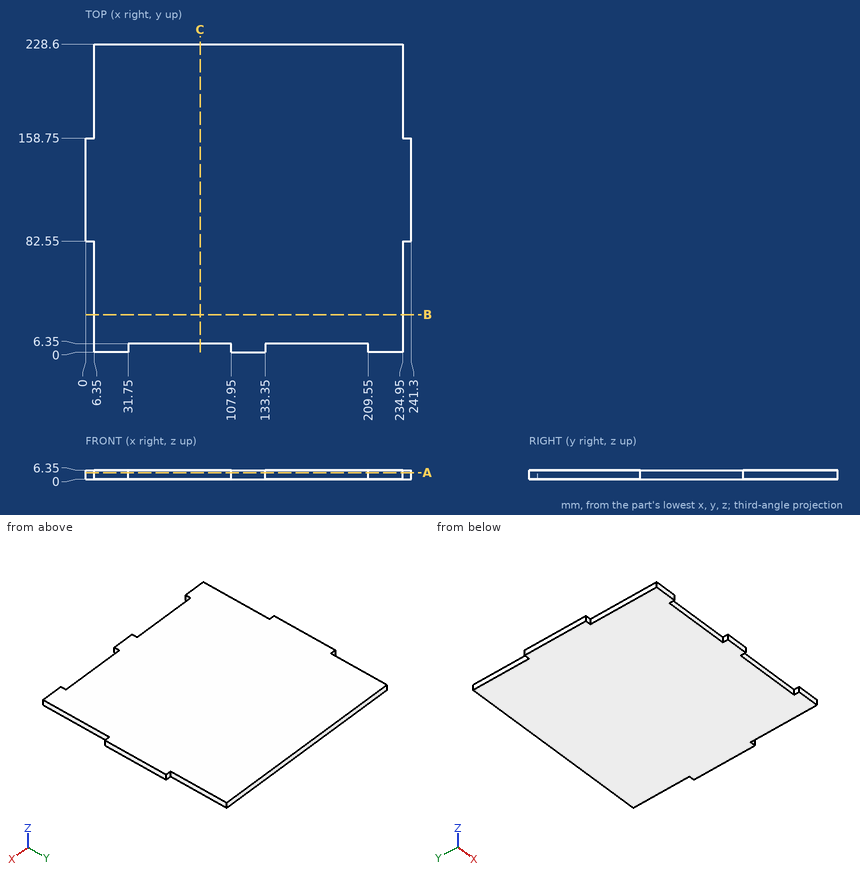
Print and shaded views of the part. All mm, measured from the part's lowest x, y and z. Coordinates: 2 decimals unless noted, no trailing zeros. Order: outer loops, then holes, each group sorted by start corner. A loop starts at its lowest first (then second) coordinate and runs counter-clockwise, first axis right, second up.
Item 1: Saw through at B-B on y = 28. List the corners of the cut face in (x, z).
Filled in:
outline: (6.35, 0) - (234.95, 0) - (234.95, 6.35) - (6.35, 6.35) - close
Item 2: Saw through at C-C on x = 85. List the corners of the cut face in (y, z), then the cut area to 3 significant figures.
Filled in:
outline: (6.35, 0) - (228.6, 0) - (228.6, 6.35) - (6.35, 6.35) - close
area: 1,410 mm2
Item 3: Drill centre lines: L1, parallel to Y at x = 52, z = 5.5; L2, parallel to X at y = 50, z = 2.5. Where is each one in solid material? Low to high.
Filled in:
L1: y = 6.35 to 228.6
L2: x = 6.35 to 234.95
Item 4: Saw through at A-A on z = 4.75. List the corners of the cut face in (x, y), then the cut area to 3 significant figures.
Filled in:
outline: (0, 82.55) - (6.35, 82.55) - (6.35, 0) - (31.75, 0) - (31.75, 6.35) - (107.95, 6.35) - (107.95, 0) - (133.35, 0) - (133.35, 6.35) - (209.55, 6.35) - (209.55, 0) - (234.95, 0) - (234.95, 82.55) - (241.3, 82.55) - (241.3, 158.75) - (234.95, 158.75) - (234.95, 228.6) - (6.35, 228.6) - (6.35, 158.75) - (0, 158.75) - close
area: 52,300 mm2
Item 5: Drop flat-ended pins along their axis: pin 1 Ø1.9 at (x, z) = (60, 4.5) entering from -Y; pin 2 Ø3 at (y, z) = (207.5, 4) entering from +X; pin 3 Ø1.9 at (y, z) = (3.5, 3.5) entering from -X. Give the stop position or say it passes through.
Filled in:
pin 1: stops at y = 6.35
pin 2: stops at x = 234.95
pin 3: stops at x = 6.35
